from build123d import *

# Parameters (mm, degrees)
SKETCH1_W           = 120
SKETCH1_H           = 41
BOSS_EXTRUDE1_DEPTH = 12.5
SKETCH2_R           = 5.2
BOSS_EXTRUDE2_DEPTH = 1.15
SKETCH3_R           = 4
BOSS_EXTRUDE3_DEPTH = 8.55
SKETCH4_R           = 4.7
BOSS_EXTRUDE4_DEPTH = 4.3
BOSS_EXTRUDE4_TAPER = 17
FILLET1_R           = 0.8
SHELL1_T            = -0.5


with BuildPart() as part:
    # Sketch1 → Boss-Extrude1 (new body)
    with BuildSketch(Plane(origin=(0, 0, 0), x_dir=(1, 0, 0), z_dir=(0, 1, 0))):
        Rectangle(SKETCH1_W, SKETCH1_H)
    extrude(amount=BOSS_EXTRUDE1_DEPTH)

    # Sketch2 → Boss-Extrude2 (add)
    with BuildSketch(Plane.XY.offset(20.5)):
        with Locations(Location((53, 6.25, 0), (0, 0, 180))):
            Circle(SKETCH2_R)
    boss_extrude2 = extrude(amount=BOSS_EXTRUDE2_DEPTH)

    # Sketch3 → Boss-Extrude3 (add)
    with BuildSketch(Plane.XY.offset(21.65)):
        with Locations((53, 6.25)):
            Circle(SKETCH3_R)
    boss_extrude3 = extrude(amount=BOSS_EXTRUDE3_DEPTH)

    # Sketch4 → Boss-Extrude4 (add)
    with BuildSketch(Plane.XY.offset(30.2)):
        with Locations((53, 6.25)):
            Circle(SKETCH4_R)
    boss_extrude4 = extrude(amount=BOSS_EXTRUDE4_DEPTH, taper=BOSS_EXTRUDE4_TAPER)

    # Mirror1: Boss-Extrude2, Boss-Extrude3, Boss-Extrude4 across plane
    add(boss_extrude2.mirror(Plane(origin=(0, 0, 0), x_dir=(0, 0, 1), z_dir=(1, 0, 0))))
    add(boss_extrude3.mirror(Plane(origin=(0, 0, 0), x_dir=(0, 0, 1), z_dir=(1, 0, 0))))
    add(boss_extrude4.mirror(Plane(origin=(0, 0, 0), x_dir=(0, 0, 1), z_dir=(1, 0, 0))))

    # Fillet1
    fillet1_edges = [part.edges().sort_by_distance(p)[0] for p in [
        (0, 12.5, -20.5),
        (0, 0, -20.5),
        (0, 0, 20.5),
        (0, 12.5, 20.5),
    ]]
    fillet(fillet1_edges, radius=FILLET1_R)

    # Shell1
    shell1_openings = [part.faces().sort_by_distance(p)[0] for p in [
        (53, 6.25, 34.5),
        (-53, 6.25, 34.5),
    ]]
    offset(amount=SHELL1_T, openings=shell1_openings, kind=Kind.INTERSECTION)


solid = part.part
Check sheet for the modelled part. Datum: model origin and axes. Units: mm. A direction names the side the tool comes from. Round coordinates to 2 decimals unless told otherwise and drop trailing zeros. Order: outer loops, then holes, each group sorted by start corner. A loop starts at its lowest first (then second) coordinate and runs counter-clockwise, first axis right, second up.
(1) Scan lines: probe 1 along X at (y, z) = (9.5, -13); probe 2 along Z at (x, y) = (-40.5, 9.5); probe 3 along Y at (x, z) = (53, 20.7). Record each from-to range of solid material in increasing order.
(2) Cross-section at A-A, the plane z = -6. Enter the section's corners in (x, y).
(3) Cross-section at B-B, the plane x = 37. Enter the section's corners in (y, z).
(4) Draft check along X on faces 4 (the flat face through (-1, 6, -20.5)), 5 (the flat face through (60, 6, 0)), 6 (the cylindrical face through (-49.503, 6.404, 25.858)). Enter one of: pulls with the +X half, pulls with the -X half, needs draft (parallel to the pull), parting line crosses it, or undercut.
(5) Go/stop test with flat-tipped pins: P1, Ø1, axis at x = 28.5, y = 5.5, coming from the +Z side; P2, Ø2.5, axis at x = 51.5, y = 5, coming from the +Z side. Record where each tip stops, or that it passes through.
(6) Access from +Z, -Z, +X, -X, +Y, -Y to the whole of each face (thin tool, end or side, straight path). Record for faces 1 (the flat face through (-1, 12.5, 0)), 2 (the cylindrical face through (57.695, 6.043, 20.567)), 3 (the cylindrical face through (-58.195, 6.021, 21.067)).
Check sheet entries:
1. probe 1: x = -60 to -59.5, 59.5 to 60
1. probe 2: z = -20.5 to -20, 20 to 20.5
1. probe 3: y = 1.05 to 1.55, 10.95 to 11.45
2. outline: (-60, 0) - (60, 0) - (60, 12.5) - (-60, 12.5) - close; hole (-59.5, 0.5) - (59.5, 0.5) - (59.5, 12) - (-59.5, 12) - close
3. outline: (0, -19.7) arc R0.8 ccw to (0.8, -20.5) - (11.7, -20.5) arc R0.8 ccw to (12.5, -19.7) - (12.5, 19.7) arc R0.8 ccw to (11.7, 20.5) - (0.8, 20.5) arc R0.8 ccw to (0, 19.7) - close; hole (0.5, -19.7) arc R0.3 ccw to (0.8, -20) - (11.7, -20) arc R0.3 ccw to (12, -19.7) - (12, 19.7) arc R0.3 ccw to (11.7, 20) - (0.8, 20) arc R0.3 ccw to (0.5, 19.7) - close
4. face 4: needs draft
4. face 5: pulls with the +X half
4. face 6: undercut
5. P1: stops at z = 20.5
5. P2: stops at z = 34.5
6. face 1: +Z, -Z, +X, -X, +Y
6. face 2: none
6. face 3: +Z
